Verification items for the finished model (mm, model axes). A direction names the side the tool comes from. Round coordinates to 2 decimals unless told otherwise and drop trailing zeros. Order: outer loops, then holes, each group sorted by start corner. A loop starts at its lowest first (then second) coordinate and runs counter-clockwise, first axis right, second up. Notation, with made-up numbers: (-19, 47.5) -> (25, 47.5) arc R18 ccw to (25, 63.5) -> close; hole circle Ø2 at (65, 62). An arc over 180 degrees is marked (long way). Return JSON: item names as keys, results as strings. Group by question number.
Item 1: Sectioned sample at A-A on x = 0. Record the cut outline in (y, z).
Item 2: Sectioned sample at B-B on y = -3. Record the cut outline in (x, z).
Item 3: Depth check by flat-ended pin: pin 1 Ø5 at (y, z) = (0, 10.5) entering from +X; pin 2 Ø8.5 at (y, z) = (-0.5, 13.5) entering from -X; pin 3 Ø2.5 at (x, y) = (-1, 2) entering from -Z. Enter the tip coordinate at first touch or a pass-through.
Item 4: Draft check along X on faces 6 (the cylindrical face through (0, 8, 19)), 7 (the cylindrical face through (0.59, 4.46, 14.79)), 8 (the flat face through (6, 0, 19)), 9 (the flat face through (0, 0, 75)). Enter one of: pulls with the +X half, pulls with the -X half, needs draft (parallel to the pull), parting line crosses it, or undercut.
Item 5: Scan lines: probe 1 along Y at (x, z) = (0, 11.25); probe 2 along Z at (x, y) = (-4.5, 7.5); probe 3 along X at (y, z) = (3.75, 36). Record each from-to range of solid material in increasing order. Write a range as from..to.
Item 6: Access from +Z, -Z, +X, -X, +Y, -Y to the whole of each face (thin tool, end or side, straight path). Record for faces 1 (the flat face through (-7, 0, 38)), 2 (the flat face through (-3, 4, 0)), 3 (the flat face through (-6, 0, 19)), 4 (the flat face through (0, 10, 56)), 5 (the cylindrical face through (0, -8, 19)).
Item 7: Sectioned sample at C-C on y = -7. Record the cut outline in (x, z), plus the area to 3 significant figures.
```python
from build123d import *

# Parameters (mm, degrees)
BOSS_EXTRUDE1_DEPTH = 38
SKETCH2_W           = 15
SKETCH2_H           = 20
BOSS_EXTRUDE2_DEPTH = 37
SKETCH3_R           = 4.5
CUT_EXTRUDE1_DEPTH  = 30


with BuildPart() as part:
    # Sketch1 → Boss-Extrude1 (new body)
    with BuildSketch(Plane.XY):
        with BuildLine():
            Line((6, -5.291502622), (6, 5.291502622))
            ThreePointArc((6, 5.291502622), (0, 8), (-6, 5.291502622))
            Line((-6, 5.291502622), (-6, -5.291502622))
            ThreePointArc((-6, -5.291502622), (0, -8), (6, -5.291502622))
        make_face()
    extrude(amount=BOSS_EXTRUDE1_DEPTH)

    # Sketch2 → Boss-Extrude2 (add)
    with BuildSketch(Plane.XY.offset(38)):
        Rectangle(SKETCH2_W, SKETCH2_H)
    extrude(amount=BOSS_EXTRUDE2_DEPTH)

    # Sketch3 → Cut-Extrude1 (cut)
    with BuildSketch(Plane(origin=(0, 0, 0), x_dir=(-1, 0, 0), z_dir=(0, 0, -1))):
        Circle(SKETCH3_R)
    extrude(amount=-CUT_EXTRUDE1_DEPTH, mode=Mode.SUBTRACT)


solid = part.part
```
Recorded:
{
 "1": {"outline": "(-10, 38) -> (-8, 38) -> (-8, 0) -> (-4.5, 0) -> (-4.5, 30) -> (4.5, 30) -> (4.5, 0) -> (8, 0) -> (8, 38) -> (10, 38) -> (10, 75) -> (-10, 75) -> close"},
 "2": {"outline": "(-7.5, 38) -> (-6, 38) -> (-6, 0) -> (-3.35, 0) -> (-3.35, 30) -> (3.35, 30) -> (3.35, 0) -> (6, 0) -> (6, 38) -> (7.5, 38) -> (7.5, 75) -> (-7.5, 75) -> close"},
 "3": {"pin 1": "x = 6", "pin 2": "x = -6", "pin 3": "z = 30"},
 "4": {"face 6": "parting line crosses it", "face 7": "undercut", "face 8": "pulls with the +X half", "face 9": "needs draft"},
 "5": {"probe 1": "-8..-4.5, 4.5..8", "probe 2": "38..75", "probe 3": "-6..6"},
 "6": {"face 1": "-Z", "face 2": "-Z, +X, -X, +Y, -Y", "face 3": "-Z, -X, +Y, -Y", "face 4": "+Z, -Z, +X, -X, +Y", "face 5": "-Z, -Y"},
 "7": {"outline": "(-7.5, 38) -> (-3.87, 38) -> (-3.87, 0) -> (3.87, 0) -> (3.87, 38) -> (7.5, 38) -> (7.5, 75) -> (-7.5, 75) -> close", "area": "849 mm²"}
}
